Autodesk Inventor part; units mm, degrees
ref_plane "YZ Plane" through (0, 0, 0) normal (1, 0, 0) x (0, 1, 0)
ref_plane "XZ Plane" through (0, 0, 0) normal (0, 1, 0) x (-1, 0, 0)
ref_plane "XY Plane" through (0, 0, 0) normal (0, 0, 1) x (1, 0, 0)
ref_plane "Work Plane1" through (-2241.136, -81.6179, 0) normal (0, 0, 1) x (1, 0, 0)
sketch "Sketch1" plane through (-2241.136, -81.6179, 0) normal (0, 0, 1) x (1, 0, 0)
  line L0 (2006.136, 61.2134) -> (2006.136, 6.6179)
  line L1 (2006.136, 6.6179) -> (2476.136, 6.6179)
  line L2 (2476.136, 6.6179) -> (2476.136, 61.2134)
  line L3 (2476.136, 61.2134) -> (2491.136, 61.2134)
  line L4 (2491.136, 61.2134) -> (2491.136, 156.6179)
  line L5 (2491.136, 156.6179) -> (2341.136, 156.6179)
  line L6 (2341.136, 156.6179) -> (2166.136, 81.6179)
  line L7 (2166.136, 81.6179) -> (1991.136, 156.6179)
  line L8 (1991.136, 156.6179) -> (1991.136, 61.2134)
  line L9 (1991.136, 61.2134) -> (2006.136, 61.2134)
  line L10 (1991.136, 91.6179) -> (1991.136, 141.6179)
  line L11 (1991.136, 141.6179) -> (1986.136, 141.6179)
  line L12 (1986.136, 91.6179) -> (1986.136, 141.6179)
  line L13 (1991.136, 91.6179) -> (1986.136, 91.6179)
  line L14 (1991.136, 21.6179) -> (1991.136, 71.6179)
  line L15 (1991.136, 71.6179) -> (1986.136, 71.6179)
  line L16 (1986.136, 21.6179) -> (1986.136, 71.6179)
  line L17 (1991.136, 21.6179) -> (1986.136, 21.6179)
  line L18 (1986.136, 91.6179) -> (1991.136, 91.6179)
  line L19 (1991.136, 91.6179) -> (1991.136, 71.6179)
  line L20 (1991.136, 71.6179) -> (1986.136, 71.6179)
  line L21 (1986.136, 71.6179) -> (1986.136, 91.6179)
  line L22 (1991.136, 156.6179) -> (1986.136, 156.6179)
  line L23 (1986.136, 156.6179) -> (1986.136, 141.6179)
  line L24 (1986.136, 141.6179) -> (1991.136, 141.6179)
  line L25 (1991.136, 141.6179) -> (1991.136, 156.6179)
  line L26 (1986.136, 21.6179) -> (1991.136, 21.6179)
  line L27 (1991.136, 21.6179) -> (1991.136, 6.6179)
  line L28 (1991.136, 6.6179) -> (1986.136, 6.6179)
  line L29 (1986.136, 6.6179) -> (1986.136, 21.6179)
  line L30 (2006.136, 6.6179) -> (1991.136, 6.6179)
  line L31 (1991.136, 6.6179) -> (1991.136, 61.2134)
  line L32 (1991.136, 61.2134) -> (2006.136, 61.2134)
  line L33 (2006.136, 61.2134) -> (2006.136, 6.6179)
  line L34 (2496.136, 91.6179) -> (2496.136, 141.6179)
  line L35 (2496.136, 141.6179) -> (2491.136, 141.6179)
  line L36 (2491.136, 91.6179) -> (2491.136, 141.6179)
  line L37 (2496.136, 91.6179) -> (2491.136, 91.6179)
  line L38 (2496.136, 21.6179) -> (2496.136, 71.6179)
  line L39 (2496.136, 71.6179) -> (2491.136, 71.6179)
  line L40 (2491.136, 21.6179) -> (2491.136, 71.6179)
  line L41 (2496.136, 21.6179) -> (2491.136, 21.6179)
  line L42 (2491.136, 6.6179) -> (2476.136, 6.6179)
  line L43 (2476.136, 6.6179) -> (2476.136, 61.2134)
  line L44 (2476.136, 61.2134) -> (2491.136, 61.2134)
  line L45 (2491.136, 61.2134) -> (2491.136, 6.6179)
  point P0 (2241.136, 81.6179)
  point P1 (1991.136, 6.6179)
  point P2 (820.3787, 21.6179)
  point P3 (1320.3787, 21.6179)
  point P4 (820.3787, 20.4045)
  point P5 (1905.7573, 6.6179)
  point P6 (1305.3787, -34.1911)
  point P7 (820.3787, 21.6179)
  point P8 (2476.136, 6.6179)
extrude "Extrusion1" add sketch "Sketch1" along normal blind 5 contours L9 L8 L7 L6 L5 L4 L3 L2 L1 L0 | L0 L30 L27 L14 L9 | L14 L17 L16 L15 L8 | L2 L3 L40 L45 L42 | L13 L12 L11 L8 | L4 L39 L38 L41 L40 | L4 L35 L34 L37
sketch "Sketch2" plane through (-2241.136, -81.6179, 5) normal (0, 0, 1) x (1, 0, 0)
  line L0 (1991.136, 6.6179) -> (2491.136, 6.6179)
  line L1 (2491.136, 6.6179) -> (2491.136, 21.6179)
  line L2 (2491.136, 21.6179) -> (2496.136, 21.6179)
  line L3 (2496.136, 21.6179) -> (2496.136, 71.6179)
  line L4 (2496.136, 71.6179) -> (2491.136, 71.6179)
  line L5 (2491.136, 71.6179) -> (2491.136, 91.6179)
  line L6 (2491.136, 91.6179) -> (2496.136, 91.6179)
  line L7 (2496.136, 91.6179) -> (2496.136, 141.6179)
  line L8 (2496.136, 141.6179) -> (2491.136, 141.6179)
  line L9 (2491.136, 141.6179) -> (2491.136, 156.6179)
  line L10 (2491.136, 156.6179) -> (2341.136, 156.6179)
  line L11 (2341.136, 156.6179) -> (2166.136, 81.6179)
  line L12 (2166.136, 81.6179) -> (1991.136, 156.6179)
  line L13 (1991.136, 156.6179) -> (1991.136, 141.6179)
  line L14 (1991.136, 141.6179) -> (1986.136, 141.6179)
  line L15 (1986.136, 141.6179) -> (1986.136, 91.6179)
  line L16 (1986.136, 91.6179) -> (1991.136, 91.6179)
  line L17 (1991.136, 91.6179) -> (1991.136, 71.6179)
  line L18 (1991.136, 71.6179) -> (1986.136, 71.6179)
  line L19 (1986.136, 71.6179) -> (1986.136, 21.6179)
  line L20 (1986.136, 21.6179) -> (1991.136, 21.6179)
  line L21 (1991.136, 21.6179) -> (1991.136, 6.6179)
  line L22 (2371.136, 156.6179) -> (2401.136, 156.6179)
  line L23 (2401.136, 156.6179) -> (2401.136, 151.6179)
  line L24 (2401.136, 151.6179) -> (2371.136, 151.6179)
  line L25 (2371.136, 151.6179) -> (2371.136, 156.6179)
  line L26 (2431.136, 156.6179) -> (2461.136, 156.6179)
  line L27 (2461.136, 156.6179) -> (2461.136, 151.6179)
  line L28 (2461.136, 151.6179) -> (2431.136, 151.6179)
  line L29 (2431.136, 151.6179) -> (2431.136, 156.6179)
  line L30 (2166.136, 81.6179) -> (1991.136, 156.6179)
  line L31 (2037.4557, 136.7666) -> (2035.4861, 132.1708)
  line L32 (2035.4861, 132.1708) -> (2063.0604, 120.3533)
  line L33 (2063.0604, 120.3533) -> (2065.03, 124.949)
  line L34 (2092.6044, 113.1314) -> (2090.6348, 108.5357)
  line L35 (2090.6348, 108.5357) -> (2118.2091, 96.7181)
  line L36 (2118.2091, 96.7181) -> (2120.1787, 101.3138)
  line L37 (2166.136, 81.6179) -> (2166.136, 154.1179)
  line L38 (2294.8163, 136.7666) -> (2296.7859, 132.1708)
  line L39 (2296.7859, 132.1708) -> (2269.2115, 120.3533)
  line L40 (2269.2115, 120.3533) -> (2267.2419, 124.949)
  line L41 (2239.6676, 113.1314) -> (2241.6372, 108.5357)
  line L42 (2241.6372, 108.5357) -> (2214.0628, 96.7181)
  line L43 (2214.0628, 96.7181) -> (2212.0932, 101.3138)
  point P0 (2241.136, 81.6179)
  point P1 (2294.8163, 136.7666)
  point P2 (2267.2419, 124.949)
  point P3 (2239.6676, 113.1314)
  point P4 (2092.6044, 113.1314)
  point P5 (2037.4557, 136.7666)
  dimension "d2" = 30
  dimension "d3" = 5
  dimension "d4" = 30
  dimension "d5" = 5
  dimension "d6" = 30
  dimension "d7" = 30
  dimension "d10" = 30
  dimension "d11" = 5
  dimension "d12" = 30
  dimension "d13" = 5
  dimension "d14" = 30
  dimension "d15" = 50
extrude "Extrusion2" cut sketch "Sketch2" against normal blind 5 contours L12 L33 L32 L31 | L27 L28 L29 L10 | L12 L36 L35 L34 | L23 L24 L25 L10 | L11 L41 L42 L43 | L38 L39 L40 L11
sketch "Sketch3" plane through (-2241.136, -81.6179, 5) normal (0, 0, 1) x (1, 0, 0)
  point P0 (2241.136, 81.6179)
sketch "Sketch4" plane through (-2241.136, -81.6179, 5) normal (0, 0, 1) x (1, 0, 0)
  line L0 (2371.136, 91.6179) -> (2401.136, 91.6179)
  line L1 (2401.136, 91.6179) -> (2401.136, 86.6179)
  line L2 (2401.136, 86.6179) -> (2371.136, 86.6179)
  line L3 (2371.136, 86.6179) -> (2371.136, 91.6179)
  line L4 (2214.0628, 96.7181) -> (2212.0932, 101.3138)
  line L5 (2212.0932, 101.3138) -> (2166.136, 81.6179)
  line L6 (2166.136, 81.6179) -> (2120.1787, 101.3138)
  line L7 (2120.1787, 101.3138) -> (2118.2091, 96.7181)
  line L8 (2118.2091, 96.7181) -> (2090.6348, 108.5357)
  line L9 (2090.6348, 108.5357) -> (2092.6044, 113.1314)
  line L10 (2092.6044, 113.1314) -> (2065.03, 124.949)
  line L11 (2065.03, 124.949) -> (2063.0604, 120.3533)
  line L12 (2063.0604, 120.3533) -> (2035.4861, 132.1708)
  line L13 (2035.4861, 132.1708) -> (2037.4557, 136.7666)
  line L14 (2037.4557, 136.7666) -> (1991.136, 156.6179)
  line L15 (1991.136, 156.6179) -> (1991.136, 141.6179)
  line L16 (1991.136, 141.6179) -> (1986.136, 141.6179)
  line L17 (1986.136, 141.6179) -> (1986.136, 91.6179)
  line L18 (1986.136, 91.6179) -> (1991.136, 91.6179)
  line L19 (1991.136, 91.6179) -> (1991.136, 71.6179)
  line L20 (1991.136, 71.6179) -> (1986.136, 71.6179)
  line L21 (1986.136, 71.6179) -> (1986.136, 21.6179)
  line L22 (1986.136, 21.6179) -> (1991.136, 21.6179)
  line L23 (1991.136, 21.6179) -> (1991.136, 6.6179)
  line L24 (1991.136, 6.6179) -> (2491.136, 6.6179)
  line L25 (2491.136, 6.6179) -> (2491.136, 21.6179)
  line L26 (2491.136, 21.6179) -> (2496.136, 21.6179)
  line L27 (2496.136, 21.6179) -> (2496.136, 71.6179)
  line L28 (2496.136, 71.6179) -> (2491.136, 71.6179)
  line L29 (2491.136, 71.6179) -> (2491.136, 91.6179)
  line L30 (2491.136, 91.6179) -> (2496.136, 91.6179)
  line L31 (2496.136, 91.6179) -> (2496.136, 141.6179)
  line L32 (2496.136, 141.6179) -> (2491.136, 141.6179)
  line L33 (2491.136, 141.6179) -> (2491.136, 156.6179)
  line L34 (2491.136, 156.6179) -> (2461.136, 156.6179)
  line L35 (2461.136, 156.6179) -> (2461.136, 151.6179)
  line L36 (2461.136, 151.6179) -> (2431.136, 151.6179)
  line L37 (2431.136, 151.6179) -> (2431.136, 156.6179)
  line L38 (2431.136, 156.6179) -> (2401.136, 156.6179)
  line L39 (2401.136, 156.6179) -> (2401.136, 151.6179)
  line L40 (2401.136, 151.6179) -> (2371.136, 151.6179)
  line L41 (2371.136, 151.6179) -> (2371.136, 156.6179)
  line L42 (2371.136, 156.6179) -> (2341.136, 156.6179)
  line L43 (2341.136, 156.6179) -> (2294.8163, 136.7666)
  line L44 (2294.8163, 136.7666) -> (2296.7859, 132.1708)
  line L45 (2296.7859, 132.1708) -> (2269.2115, 120.3533)
  line L46 (2269.2115, 120.3533) -> (2267.2419, 124.949)
  line L47 (2267.2419, 124.949) -> (2239.6676, 113.1314)
  line L48 (2239.6676, 113.1314) -> (2241.6372, 108.5357)
  line L49 (2241.6372, 108.5357) -> (2214.0628, 96.7181)
  line L50 (2431.136, 91.6179) -> (2461.136, 91.6179)
  line L51 (2461.136, 91.6179) -> (2461.136, 86.6179)
  line L52 (2461.136, 86.6179) -> (2431.136, 86.6179)
  line L53 (2431.136, 86.6179) -> (2431.136, 91.6179)
  point P0 (2241.136, 81.6179)
  dimension "d16" = 30
  dimension "d17" = 5
  dimension "d18" = 80
  dimension "d19" = 30
  dimension "d20" = 5
  dimension "d21" = 30
  dimension "d22" = 30
extrude "Extrusion3" cut sketch "Sketch4" against normal blind 5 contours L0 L1 L2 L3 | L50 L51 L52 L53
properties part number "Frontal"
The model under review builds one solid part; all positions refer to its coordinate system, in mm. A direction names the side the tool comes from. Give positions to 0.01 mm unless a question says otherwise; leave off trailing zeros. Loops run counter-clockwise (first coordinate to the right, second up) from the corner with the lowest first, then second, coordinate; pieces in that order, holes last. Notation, with made-up numbers: (-40, 57) -> (-32, 57) arc R11 cw to (-32, 72) -> close; hole circle Ø4 at (67, -24.5). An arc over 180 degrees is marked (long way). Put each result on its own line as item: value. Start each with the question number.
1. Wall thickness on probe 1 along X at (y, z) = (40.5, 1.5); probe 2 along X at (y, z) = (40, 3.9); probe 3 along X at (y, z) = (-63, 1.2): over which ranges is each line inside the solid? List them lowest first.
2. Clearance check with flat-ended pins moving along their axes: P1, Ø1.5, axis at x = 199.5, z = 2.5, coming from the +Y side; P2, Ø2.5, axis at y = 69, z = 2.5, coming from the +X side; P3, Ø1.5, axis at x = 187.5, y = -30, coming from the -Z side; P4, Ø1.5, axis at y = 6.5, z = 2, coming from the -X side. State where each tip first meets the part, or that it passes through.
3. For faces 1 (the face through (-4, -16, 5)), 2 (the face through (-226.516, 64.935, 2.465)), list the 3-axis set-ups (+Z, -Z, +X, -X, +Y, -Y) from which the entire face can be reached by the end or side of a thin tool; tool diameter is ignored.
4. We need section C-C on x = -101. State the section outline as (y, z) points, then the cut area to 3 significant figures.
5. We need section B-B on x = -44.5. State the section outline as (y, z) points, then the cut area to 3 significant figures.
6. We need section A-A on z = 1.5. State how many separate pieces and enclosed holes the cut face has, then the cut area to 3 significant figures.
Determined:
1. probe 1: -255 to -182.19, -177.32 to -169.5, 19.5 to 27.32, 32.19 to 255
1. probe 2: -255 to -181.03, -177.53 to -168.33, 18.33 to 27.53, 31.03 to 255
1. probe 3: -250 to 250
2. P1: y = 70
2. P2: x = 250
2. P3: z = 0
2. P4: x = -250
3. face 1: +Z, +X, -X, +Y, -Y
3. face 2: +Z, -Z, +Y
4. outline: (-75, 0) -> (11.14, 0) -> (11.14, 5) -> (-75, 5) -> close
4. area: 431 mm^2
5. outline: (-75, 0) -> (13.07, 0) -> (13.07, 5) -> (-75, 5) -> close
5. area: 440 mm^2
6. separate pieces: 1
6. enclosed holes: 2
6. area: 61,700 mm^2
